from build123d import *

# Parameters (mm, degrees)
SKETCH2_W           = 45
SKETCH2_H           = 35
BOSS_EXTRUDE1_DEPTH = 10
SKETCH3_W           = 20
SKETCH3_H           = 20
CUT_EXTRUDE1_DEPTH  = 2
SKETCH10_R          = 2.85
CUT_EXTRUDE2_DEPTH  = 7


with BuildPart() as part:
    # Sketch2 → Boss-Extrude1 (new body)
    with BuildSketch(Plane(origin=(0, 0, 0), x_dir=(1, 0, 0), z_dir=(0, 1, 0))):
        Rectangle(SKETCH2_W, SKETCH2_H)
    extrude(amount=BOSS_EXTRUDE1_DEPTH)

    # Sketch3 → Cut-Extrude1 (cut)
    with BuildSketch(Plane(origin=(0, 10, 0), x_dir=(1, 0, 0), z_dir=(0, 1, 0))):
        Rectangle(SKETCH3_W, SKETCH3_H)
    extrude(amount=-CUT_EXTRUDE1_DEPTH, mode=Mode.SUBTRACT)

    # Sketch10 → Cut-Extrude2 (cut)
    with BuildSketch(Plane.XZ):
        with Locations(Location((-18.75, 13.75, 0), (0, 0, 270))):
            Circle(SKETCH10_R)
        with Locations(Location((18.754391979, 13.75, 0), (0, 0, 270))):
            Circle(SKETCH10_R)
        with Locations(Location((18.754391979, -13.75, 0), (0, 0, 270))):
            Circle(SKETCH10_R)
        with Locations(Location((-18.75, -13.75, 0), (0, 0, 270))):
            Circle(SKETCH10_R)
    extrude(amount=-CUT_EXTRUDE2_DEPTH, mode=Mode.SUBTRACT)


solid = part.part
Geometry: final body of the model. Coordinates: model frame, mm. A direction names the side the tool comes from. Round coordinates to 2 decimals unless told otherwise and drop trailing zeros. Loops run counter-clockwise (first coordinate to the right, second up) from the corner with the lowest first, then second, coordinate; pieces in that order, holes last.
Q1. Access query for faces 1 (the flat face through (0, 9, 10)), 2 (the flat face through (0, 5, -17.5)), 3 (the flat face through (-19, 7, -14)). Directions: +Z, -Z, +X, -X, +Y, -Y. A direction counts if a zero-diameter tool reaches every point of the face in a straight line with its end or side. Return the directions, or none.
Q2. Pull-direction query (X, two-part tool) for faces 4 (the flat face through (0, 5, 17.5)), 5 (the flat face through (-10, 9, 0)), 6 (the flat face through (-22.5, 5, 0)); classes: released by +X, released by -X, zero draft, split by the parting line, or undercut.
Q3. Pin query (flat end, axial travel): P1, Ø4.5, axis at x = 19.5, z = 15, coming from the -Y side; P2, Ø3, axis at x = -19.5, z = 13, coming from the -Y side. Return the tip coordinate at first contact, or that it passes through.
Q4. Material intervals for L1, parallel to X at y = 5, z = -13.75; L2, parallel to Z at x = 18.5, y = 2.75; L3, parallel to Z at x = 8, y = 9, sorted ascending.
Q5. Section A-A on x = -18.75. Return loops of the section in (y, z), plus the area to 3 significant figures.
Q6. Section D-D on x = -3.5. Return loops of the section in (y, z), plus the area to 3 significant figures.
Q7. Section C-C on z = 13.75. Return loops of the section in (x, y).
Q8. Section B-B on y = 2.5. Return loops of the section in (x, z), plus the area to 3 significant figures.
Evaluation:
1. face 1: +Y
1. face 2: -Z, +X, -X, +Y, -Y
1. face 3: -Y
2. face 4: zero draft
2. face 5: undercut
2. face 6: released by -X
3. P1: stops at y = 0
3. P2: stops at y = 7
4. L1: x = -22.5 to -21.6, -15.9 to 15.9, 21.6 to 22.5
4. L2: z = -17.5 to -16.59, -10.91 to 10.91, 16.59 to 17.5
4. L3: z = -17.5 to -10, 10 to 17.5
5. outline: (0, -17.5) - (10, -17.5) - (10, 17.5) - (0, 17.5) - (0, 16.6) - (7, 16.6) - (7, 10.9) - (0, 10.9) - (0, -10.9) - (7, -10.9) - (7, -16.6) - (0, -16.6) - close
5. area: 270 mm2
6. outline: (0, -17.5) - (10, -17.5) - (10, -10) - (8, -10) - (8, 10) - (10, 10) - (10, 17.5) - (0, 17.5) - close
6. area: 310 mm2
7. outline: (-22.5, 0) - (-21.6, 0) - (-21.6, 7) - (-15.9, 7) - (-15.9, 0) - (15.9, 0) - (15.9, 7) - (21.6, 7) - (21.6, 0) - (22.5, 0) - (22.5, 10) - (-22.5, 10) - close
8. outline: (-22.5, -17.5) - (22.5, -17.5) - (22.5, 17.5) - (-22.5, 17.5) - close; hole circle Ø5.7 at (-18.75, -13.75); hole circle Ø5.7 at (-18.75, 13.75); hole circle Ø5.7 at (18.75, -13.75); hole circle Ø5.7 at (18.75, 13.75)
8. area: 1,470 mm2
